Geometry: final body of the model. Coordinates: model frame, mm. A direction names the side the tool comes from. Give positions to 0.01 mm unless a question says otherwise; leave off trailing zeros. Write each loop counter-clockwise with the first axis right and the second up, starting at its lowest first coordinate (ties: lowest second). Pieces come first, ordered by that corner, then holes.
from build123d import *

# Parameters (mm, degrees)
SKETCH1_W           = 15
SKETCH1_H           = 25.4
BOSS_EXTRUDE1_DEPTH = 3.175
SKETCH2_W           = 15
SKETCH2_H           = 3.175
BOSS_EXTRUDE2_DEPTH = 22.225
SKETCH4_R           = 1.5
CUT_EXTRUDE3_DEPTH  = 37.933868265
SKETCH3_R           = 1.5
CUT_EXTRUDE4_DEPTH  = 39.927111375
SKETCH5_W           = 22.225
SKETCH5_H           = 15
CUT_EXTRUDE5_DEPTH  = 1.5875
CUT_EXTRUDE6_START  = -1.5875
SKETCH6_W           = 15
SKETCH6_H           = 23.8125
CUT_EXTRUDE6_DEPTH  = 1.5875
SKETCH7_W           = 23.8125
SKETCH7_H           = 15
SKETCH7_R           = 1.5
BOSS_EXTRUDE5_DEPTH = 1.585
BOSS_EXTRUDE6_START = 1.585
SKETCH8_W           = 14.97890093
SKETCH8_H           = 22.2275
SKETCH8_R           = 1.5
BOSS_EXTRUDE6_DEPTH = 1.585


with BuildPart() as part:
    # Sketch1 → Boss-Extrude1 (new body)
    with BuildSketch(Plane(origin=(0, 0, 0), x_dir=(0, 0, -1), z_dir=(1, 0, 0))):
        with Locations((7.5, 12.7)):
            Rectangle(SKETCH1_W, SKETCH1_H)
    extrude(amount=BOSS_EXTRUDE1_DEPTH)

    # Sketch2 → Boss-Extrude2 (add)
    with BuildSketch(Plane(origin=(3.175, 0, 0), x_dir=(0, 0, -1), z_dir=(1, 0, 0))):
        with Locations((7.5, 1.5875)):
            Rectangle(SKETCH2_W, SKETCH2_H)
    extrude(amount=BOSS_EXTRUDE2_DEPTH)

    # Sketch4 → Cut-Extrude3 (cut, through all)
    with BuildSketch(Plane(origin=(3.175, 0, 0), x_dir=(0, 0, -1), z_dir=(1, 0, 0))):
        with Locations((7.5, 17.9)):
            Circle(SKETCH4_R)
        with Locations((7.5, 10.4)):
            Circle(SKETCH4_R)
    extrude(amount=-CUT_EXTRUDE3_DEPTH, mode=Mode.SUBTRACT)

    # Sketch3 → Cut-Extrude4 (cut, through all)
    with BuildSketch(Plane.XZ):
        with Locations(Location((10.4, -7.5, 0), (0, 0, 270))):
            Circle(SKETCH3_R)
        with Locations(Location((17.9, -7.5, 0), (0, 0, 270))):
            Circle(SKETCH3_R)
    extrude(amount=-CUT_EXTRUDE4_DEPTH, mode=Mode.SUBTRACT)

    # Sketch5 → Cut-Extrude5 (cut)
    with BuildSketch(Plane(origin=(0, 3.175, 0), x_dir=(1, 0, 0), z_dir=(0, 1, 0))):
        with Locations((14.2875, 7.5)):
            Rectangle(SKETCH5_W, SKETCH5_H)
    extrude(amount=-CUT_EXTRUDE5_DEPTH, mode=Mode.SUBTRACT)

    # Sketch6 → Cut-Extrude6 (cut)
    with BuildSketch(Plane(origin=(3.175, 0, 0), x_dir=(0, 0, -1), z_dir=(1, 0, 0)).offset(CUT_EXTRUDE6_START)):
        with Locations((7.5, 13.49375)):
            Rectangle(SKETCH6_W, SKETCH6_H)
    extrude(amount=CUT_EXTRUDE6_DEPTH, mode=Mode.SUBTRACT)

    # Sketch7 → Boss-Extrude5 (add)
    with BuildSketch(Plane(origin=(0, 1.5875, 0), x_dir=(1, 0, 0), z_dir=(0, 1, 0))):
        with Locations((13.49375, 7.5)):
            Rectangle(SKETCH7_W, SKETCH7_H)
        with Locations(Location((10.4, 7.5, 0), (0, 0, 90))):
            Circle(SKETCH7_R, mode=Mode.SUBTRACT)
        with Locations(Location((17.9, 7.5, 0), (0, 0, 90))):
            Circle(SKETCH7_R, mode=Mode.SUBTRACT)
    extrude(amount=BOSS_EXTRUDE5_DEPTH)

    # Sketch8 → Boss-Extrude6 (add)
    with BuildSketch(Plane(origin=(1.5875, 0, 0), x_dir=(0, 0, -1), z_dir=(1, 0, 0)).offset(BOSS_EXTRUDE6_START)):
        with Locations((7.489450465, 14.28625)):
            Rectangle(SKETCH8_W, SKETCH8_H)
        with Locations((7.5, 17.9)):
            Circle(SKETCH8_R, mode=Mode.SUBTRACT)
        with Locations((7.5, 10.4)):
            Circle(SKETCH8_R, mode=Mode.SUBTRACT)
    extrude(amount=-BOSS_EXTRUDE6_DEPTH)


solid = part.part
Q1. Section B-B on z = -7.5. Output: boundary loops of the cut face in (x, y).
Filled sheet:
outline: (0, 0) - (8.9, 0) - (8.9, 3.17) - (3.17, 3.17) - (3.17, 8.9) - (0, 8.9) - close; (0, 11.9) - (3.17, 11.9) - (3.17, 16.4) - (0, 16.4) - close; (0, 19.4) - (3.17, 19.4) - (3.17, 25.4) - (0, 25.4) - close; (11.9, 0) - (16.4, 0) - (16.4, 3.17) - (11.9, 3.17) - close; (19.4, 0) - (25.4, 0) - (25.4, 3.17) - (19.4, 3.17) - close
Q2. Access query for faces 1 (the cylindrical face through (1.61, 11.41, -6.39)), 2 (the flat face through (3.172, 14, -7)). Directions: +Z, -Z, +X, -X, +Y, -Y. A direction counts if a zero-diameter tool reaches every point of the face in a straight line with its end or side. Return the directions, or none.
Filled sheet:
face 1: +X, -X
face 2: +Z, -Z, +X, +Y
Q3. Ray query, line 1 along X through (y, z) = (2.15, -7.5); line 2 along Z through (x, y) = (10.4, 1.6). Return the intervals inside material, ascending.
Filled sheet:
line 1: x = 0 to 8.9, 11.9 to 16.4, 19.4 to 25.4
line 2: z = -15 to -9, -6 to 0
Q4. Pin query (flat end, axial travel): P1, Ø1.5, axis at x = 12.5, z = -5, coming from the +Y side; P2, Ø1.5, axis at x = 17.5, z = -6.5, coming from the -Y side; P3, Ø1, axis at y = 12, z = -2, coming from the +X side; P4, Ø0.5, axis at x = 2, y = 15, coming from the -Z side. Return the tip coordinate at first contact, or that it passes through.
Filled sheet:
P1: stops at y = 3.17
P2: stops at y = 0
P3: stops at x = 3.17
P4: stops at z = -14.98
Q5. Pull-direction query (X, two-part tool) for faces 3 (the flat face through (7, 2, -15)), 4 (the cylindrical face through (16.89, 1.56, -6.39)), 5 (the flat face through (0, 13, -7)), 6 (the cylindrical face through (9.39, 1.56, -6.39)); classes: released by +X, released by -X, zero draft, split by the parting line, or undercut.
Filled sheet:
face 3: zero draft
face 4: undercut
face 5: released by -X
face 6: undercut
Q6. Section C-C on x = 17.9. Output: boundary loops of the cut face in (y, z), plus the area to 3 significant figures.
Filled sheet:
outline: (0, -15) - (3.17, -15) - (3.17, -9) - (0, -9) - close; (0, -6) - (3.17, -6) - (3.17, 0) - (0, 0) - close
area: 38.1 mm2
